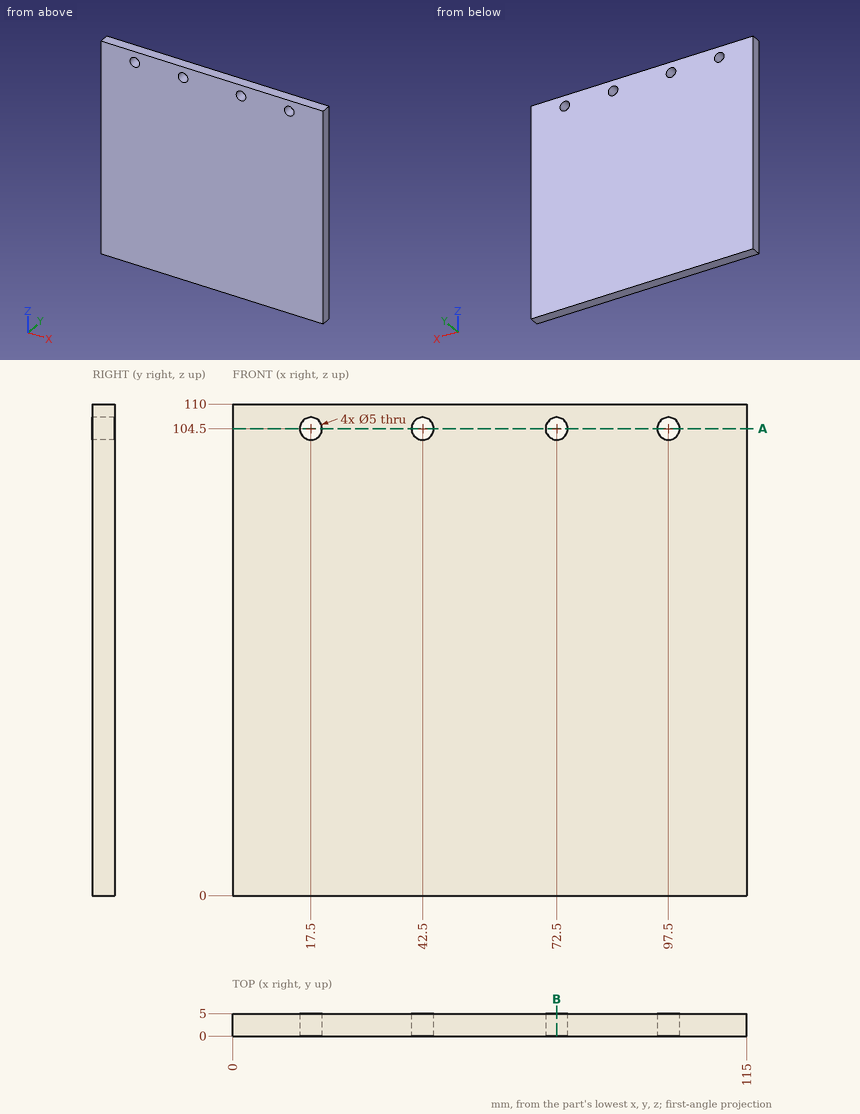
Input: dimensioned drawing with shaded views. Units: mm. Origin: part minimum x, y, z. Round coordinates to 2 decimals unless told otherwise and drop trailing zeros. Write each loop counter-clockwise with the first axis right and the second up, starting at its lowest first coordinate (ties: lowest second). Pieces come first, ordered by that corner, then holes. Notation, with made-up numbers: (15, 84.5) - (52, 84.5) arc R12 ccw to (52, 100.5) - close; hole circle Ø3 at (0.25, 24.25). An arc over 180 degrees is marked (long way). Write item = value, one per line.
(1) Section query A-A on z = 104.5. Output: boundary loops of the cut face in (x, y), then the cut area to 3 significant figures.
Geometry check:
outline = (0, 0) - (15, 0) - (15, 5) - (0, 5) - close; (20, 0) - (40, 0) - (40, 5) - (20, 5) - close; (45, 0) - (70, 0) - (70, 5) - (45, 5) - close; (75, 0) - (95, 0) - (95, 5) - (75, 5) - close; (100, 0) - (115, 0) - (115, 5) - (100, 5) - close
area = 475 mm^2
(2) Section query B-B on x = 72.5. Output: boundary loops of the cut face in (y, z).
Geometry check:
outline = (0, 0) - (5, 0) - (5, 102) - (0, 102) - close; (0, 107) - (5, 107) - (5, 110) - (0, 110) - close
(3) Material intervals for probe 1 along X at (y, z) = (2.15, 104.5); probe 2 along Z at (x, y) = (72.5, 1.85); probe 3 along Z at (x, y) = (18, 4.6), sorted ascending.
Geometry check:
probe_1 = 0 to 15, 20 to 40, 45 to 70, 75 to 95, 100 to 115
probe_2 = 0 to 102, 107 to 110
probe_3 = 0 to 102.05, 106.95 to 110
